```python
from build123d import *

# Parameters (mm, degrees)
BOSS_EXTRUDE1_DEPTH = 26
CHAMFER1_SIZE       = 10


with BuildPart() as part:
    # Sketch1 → Boss-Extrude1 (new body)
    with BuildSketch(Plane(origin=(0, 0, 0), x_dir=(0, 0, -1), z_dir=(1, 0, 0))):
        Polygon((0, 0), (0, 70.000000066), (16, 70.000000066), (16, 15.000000066), (112, 15.000000066), (112, 70.000000066), (128, 70.000000066), (128, 0), align=None)
    extrude(amount=BOSS_EXTRUDE1_DEPTH)

    # Chamfer1
    chamfer1_edges = [part.edges().sort_by_distance(p)[0] for p in [
        (13, 15.000000066, -16),
        (13, 15.000000066, -112),
    ]]
    chamfer(chamfer1_edges, length=CHAMFER1_SIZE)


solid = part.part
```
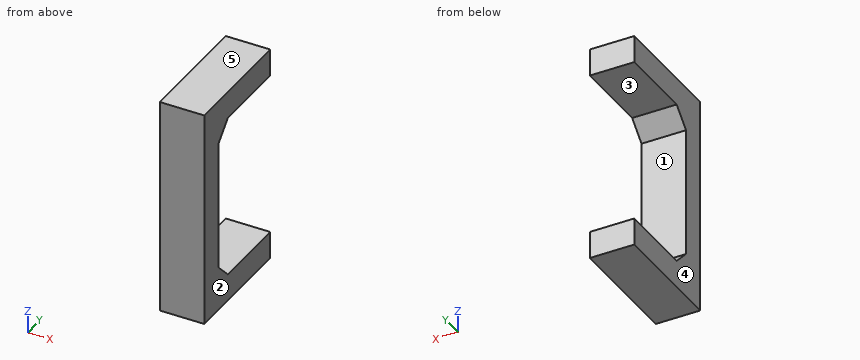
For this review, take the finished solid that the model builds, in its own axes (mm). Face numbers are marked on the shaded views. A direction names the side the tool comes from. Give positions to 0.01 mm unless a question says otherwise; leave off trailing zeros. Write each loop counter-clockwise with the first axis right and the second up, starting at its lowest first coordinate (ties: lowest second). Pieces come first, ordered by that corner, then holes.
Item 1: Take a section at A-A (y = 20). Give the boundary of the cut face in (x, z), and give its area (3 significant figures).
Item 2: Wall thickness on probe 1 along Z at (x, y) = (19.25, 64.5); probe 2 along Y at (x, z) = (15.5, -88); probe 3 along Z at (x, y) = (8.75, 19): over which ranges is each line inside the solid? List them lowest first.
Item 3: Take a section at B-B (x = 7.5). Give the boundary of the cut face in (y, z), and give its area (3 significant figures).
Item 4: Insertion check: P1, Ø6, axis at x = 10.5, z = -94.5, coming from the +Y side; P2, Ø8, axis at x = 16, z = -102.5, coming from the +Y side. Each pin has a flat end and moves straight along its axis. Give the tip position at first contact, or say it passes through.
Item 5: Machinability: for the marked faces 1 and 2, which of the approach directions +Z, -Z, +X, -X, +Y, -Y give a long, thin tool a straight path to every point of the face, cutting with its end or side? Answer none if there is none.
Item 6: Take a section at D-D (z = -106). Give the boundary of the cut face in (x, y), and give its area (3 significant figures).
Item 7: The part is to be moulded in two halves that separate along Z. For the marked faces 3, 4 and 5, say which applies: +Z half, -Z half, draft (parallel to the pull), parting line (faces both ways), or undercut.
Item 8: Take a section at C-C (y = 54). Give the boundary of the cut face in (x, z), and give its area (3 significant figures).
Established:
1. outline: (0, -128) - (26, -128) - (26, -107) - (0, -107) - close; (0, -21) - (26, -21) - (26, 0) - (0, 0) - close
1. area: 1,090 mm2
2. probe 1: z = -128 to -112, -16 to 0
2. probe 2: y = 0 to 15
2. probe 3: z = -128 to -106, -22 to 0
3. outline: (0, -128) - (70, -128) - (70, -112) - (25, -112) - (15, -102) - (15, -26) - (25, -16) - (70, -16) - (70, 0) - (0, 0) - close
3. area: 3,780 mm2
4. P1: stops at y = 15
4. P2: stops at y = 19.5
5. face 1: +X, -X, +Y
5. face 2: +Z, -Z, +X, +Y, -Y
6. outline: (0, 0) - (26, 0) - (26, 19) - (0, 19) - close
6. area: 494 mm2
7. face 3: undercut
7. face 4: draft
7. face 5: +Z half
8. outline: (0, -128) - (26, -128) - (26, -112) - (0, -112) - close; (0, -16) - (26, -16) - (26, 0) - (0, 0) - close
8. area: 832 mm2
